Here's how the part is built. I have some questions about the finished solid (model axes, mm). Face numbers are marked on the shaded views. A direction names the side the tool comes from. Coordinates: 2 decimals unless noted, no trailing zeros. Order: outer loops, then holes, each group sorted by start corner. A loop starts at its lowest first (then second) coordinate and runs counter-clockwise, first axis right, second up. Notation, with made-up numbers: M 7.5,11.5 L 51.5,11.5 A14 cw 51.5,24.5 Z; hole C 60,-12 d6. An arc over 180 degrees is marked long. One line per question, with ' | ' between items. Start each with the question number.
```python
from build123d import *

# Parameters (mm, degrees)
F0_W     = 40
F0_H     = 21
F1_DEPTH = 4
F2_W     = 37.5
F2_H     = 17.2
F3_DEPTH = 10
F4_SIZE  = 5
F5_R     = 0.5
F6_SIZE  = 0.5


with BuildPart() as f1:
    # F0 (on Top) → F1 (new body)
    with BuildSketch(Plane.XY):
        Rectangle(F0_W, F0_H)
    extrude(amount=F1_DEPTH)

    # F2 (on face) → F3 (join)
    with BuildSketch(Plane.XY.offset(4)):
        Rectangle(F2_W, F2_H)
    extrude(amount=F3_DEPTH)

    # F4
    f4_edges = [f1.edges().sort_by_distance(p)[0] for p in [
        (18.75, -8.6, 9),
        (-18.75, -8.6, 9),
        (18.75, 8.6, 9),
        (-18.75, 8.6, 9),
    ]]
    chamfer(f4_edges, length=F4_SIZE)

    # F5
    f5_edges = [f1.edges().sort_by_distance(p)[0] for p in [
        (-20, -10.5, 2),
        (-20, 10.5, 2),
        (20, -10.5, 2),
        (20, 10.5, 2),
    ]]
    fillet(f5_edges, radius=F5_R)

    # F6
    f6_edges = [f1.edges().sort_by_distance(p)[0] for p in [
        (20, 0, 0),
    ]]
    chamfer(f6_edges, length=F6_SIZE)


solid = f1.part
```
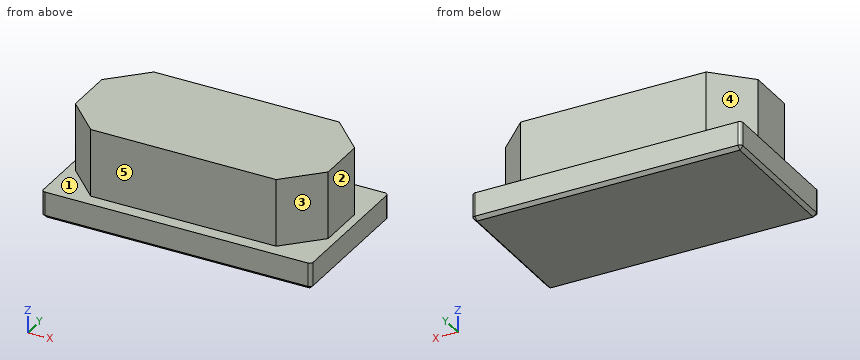
1. Will these pins go through, and if not, where does the flat tip stop? pin 1 (1.5 mm diameter, centred on y = 8, z = 12, fed in from -X); pin 2 (6 mm diameter, centred on y = -1, z = 8, fed in from +X); pin 3 (3.5 mm diameter, centred on y = -0.5, z = 8, fed in from -X).
2. I need wall thicknesses on line 1 (Y direction, x = 13, z = 9.5); line 2 (X direction, y = 3.5, z = 10.5); line 3 (X direction, y = 8.25, z = 9). Which ranges of each line are inside material? Lowest first, please.
3. Imagine slicing it at A-A (y = -7). List the corners of the cut face in (x, z) for me.
4. Imagine slicing it at C-C (z = 5.75). List the corners of the cut face in (x, y) for me, then the cut area to 3 significant figures.
5. Imagine slicing it at B-B (x = 15.5). List the corners of the cut face in (y, z) for me, then the cut area to 3 significant figures.
6. Which directions (+Z, -Z, +X, -X, +Y, -Y) give clear straight access to the entire face, cutting with the end or side of a thin tool? Please do the marked faces 1, 2, 3, 4 and 5.
7. Imagine slicing it at D-D (y = 9.25). List the corners of the cut face in (x, z) for me.
Entries:
1) pin 1: x = -15.1 | pin 2: x = 18.75 | pin 3: x = -18.75
2) line 1: -8.6 to 8.6 | line 2: -18.75 to 18.75 | line 3: -14.1 to 14.1
3) outline: M -20,0.5 L -19.5,0 L 19.5,0 L 20,0.5 L 20,4 L 15.35,4 L 15.35,14 L -15.35,14 L -15.35,4 L -20,4 Z
4) outline: M -18.75,-3.6 L -13.75,-8.6 L 13.75,-8.6 L 18.75,-3.6 L 18.75,3.6 L 13.75,8.6 L -13.75,8.6 L -18.75,3.6 Z | area: 595 mm²
5) outline: M -10.5,0.5 L -10,0 L 10,0 L 10.5,0.5 L 10.5,4 L 6.85,4 L 6.85,14 L -6.85,14 L -6.85,4 L -10.5,4 Z | area: 221 mm²
6) face 1: +Z | face 2: +Z, +X, +Y, -Y | face 3: +Z, +X, -Y | face 4: +Z, -X, +Y | face 5: +Z, +X, -X, -Y
7) outline: M -20,0.5 L -19.5,0 L 19.5,0 L 20,0.5 L 20,4 L -20,4 Z
